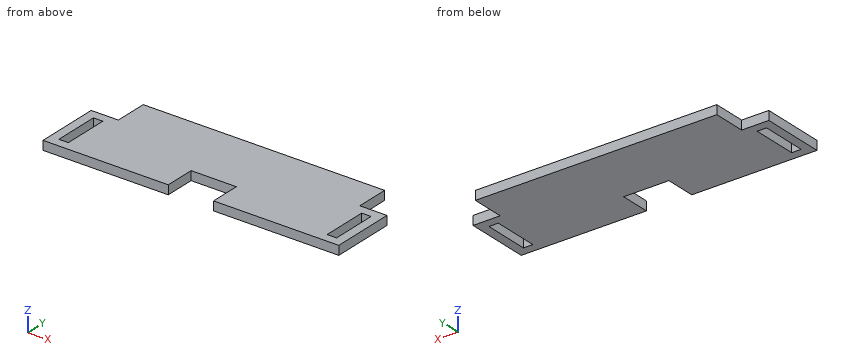
```python
from build123d import *

# Parameters (mm, degrees)
CROQUIS1_W              = 3.123
CROQUIS1_H              = 15.13
SALIENTE_EXTRUIR1_DEPTH = 3
CROQUIS2_W              = 15
CROQUIS2_H              = 10
CORTAR_EXTRUIR1_DEPTH   = 4


with BuildPart() as part:
    # Croquis1 → Saliente-Extruir1 (new body)
    with BuildSketch(Plane.XY):
        Polygon((-49, 0), (49, 0), (49, 21.123), (40, 21.123), (40, 32), (-40, 32), (-40, 21.123), (-49, 21.123), align=None)
        with Locations((-44.4385, 10.558)):
            Rectangle(CROQUIS1_W, CROQUIS1_H, mode=Mode.SUBTRACT)
        with Locations((44.4385, 10.558)):
            Rectangle(CROQUIS1_W, CROQUIS1_H, mode=Mode.SUBTRACT)
    extrude(amount=SALIENTE_EXTRUIR1_DEPTH)

    # Croquis2 → Cortar-Extruir1 (cut, through all)
    with BuildSketch(Plane.XY.offset(3)):
        with Locations((0, 5)):
            Rectangle(CROQUIS2_W, CROQUIS2_H)
    extrude(amount=-CORTAR_EXTRUIR1_DEPTH, mode=Mode.SUBTRACT)


solid = part.part
```
Source: CAD feature listing. Evaluate the final solid. Frame: model axes, mm. Coordinates: 2 decimals unless noted, no trailing zeros. Loops run counter-clockwise (first coordinate to the right, second up) from the corner with the lowest first, then second, coordinate; pieces in that order, holes last. Notation, with made-up numbers: M 7.5,26.25 L 60.5,26.25 A23 ccw 60.5,58.25 Z; hole C -31,13.25 d9. An arc over 180 degrees is marked long. Use a Markdown table: item, result. Add a question column.
Q1. Section query B-B, the plane z = 1.2. Return loops of the section in (x, y).
Q2. Material intervals for L1, parallel to X at y = 18, z = 2.2; L2, parallel to X at y = 4, z = 0.75; L3, parallel to Y at x = -6.5, z = 0.3, sorted ascending.
Q3. Section query A-A, the plane y = 12.5. Return loops of the section in (x, z).
Q4. Section query D-D, the plane x = 0.5. Return loops of the section in (y, z), and give its area (3 significant figures).
Q5. First-contact query: pin 1 (0.9 mm diameter, centred on x = 45, z = 2, fed in from +Y); pin 2 (0.9 mm diameter, centred on x = -1, z = 1, fed in from -Y); pin 3 (0.9 mm diameter, centred on y = 26.5, z = 2, fed in from +X). Flat tips, straight axial feed; report the tip coordinate or a pass-through.
Q6. Section query C-C, the plane y = 4.5. Return loops of the section in (x, z).
Result:
| question | item | result |
|---|---|---|
| 1 | outline | M -49,0 L -7.5,0 L -7.5,10 L 7.5,10 L 7.5,0 L 49,0 L 49,21.12 L 40,21.12 L 40,32 L -40,32 L -40,21.12 L -49,21.12 Z; hole M -46,2.99 L -42.88,2.99 L -42.88,18.12 L -46,18.12 Z; hole M 42.88,2.99 L 46,2.99 L 46,18.12 L 42.88,18.12 Z |
| 2 | L1 | x = -49 to -46, -42.88 to 42.88, 46 to 49 |
| 2 | L2 | x = -49 to -46, -42.88 to -7.5, 7.5 to 42.88, 46 to 49 |
| 2 | L3 | y = 10 to 32 |
| 3 | outline | M -49,0 L -46,0 L -46,3 L -49,3 Z; M -42.88,0 L 42.88,0 L 42.88,3 L -42.88,3 Z; M 46,0 L 49,0 L 49,3 L 46,3 Z |
| 4 | outline | M 10,0 L 32,0 L 32,3 L 10,3 Z |
| 4 | area | 66.0 mm2 |
| 5 | pin 1 | stops at y = 21.12 |
| 5 | pin 2 | stops at y = 10 |
| 5 | pin 3 | stops at x = 40 |
| 6 | outline | M -49,0 L -46,0 L -46,3 L -49,3 Z; M -42.88,0 L -7.5,0 L -7.5,3 L -42.88,3 Z; M 7.5,0 L 42.88,0 L 42.88,3 L 7.5,3 Z; M 46,0 L 49,0 L 49,3 L 46,3 Z |
